Can you work these out from the model? Positions are in its coordinate system, mm. A direction names the side the tool comes from. Round coordinates to 2 decimals unless told otherwise and drop trailing zeros. Loops run counter-clockwise (first coordinate to the right, second up) from the corner with the lowest first, then second, coordinate; pieces in that order, holes last. Notation, with made-up numbers: M -13.75,20 L 31.25,20 A23 cw 31.25,31 Z; hole C 89,65 d6. An arc over 180 degrees is marked long. Use a Markdown table: item, result. Add a question column.
```python
from build123d import *

# Parameters (mm, degrees)
SKETCH1_R           = 3
SKETCH1_R_2         = 1.6
BOSS_EXTRUDE1_DEPTH = 3


with BuildPart() as part:
    # Sketch1 → Boss-Extrude1 (new body)
    with BuildSketch(Plane.XY):
        Polygon((330.61212976, -150), (350.61212976, -150), (350.61212976, -193), (345.61212976, -198), (330.61212976, -198), (308.61212976, -198), (303.61212976, -193), (303.61212976, -187), (308.61212976, -182), (325.61212976, -182), (330.61212976, -177), align=None)
        with Locations((311.11212976, -187.1)):
            Circle(SKETCH1_R, mode=Mode.SUBTRACT)
        with Locations((334.61212976, -155)):
            Circle(SKETCH1_R_2, mode=Mode.SUBTRACT)
        with Locations((346.61212976, -155)):
            Circle(SKETCH1_R_2, mode=Mode.SUBTRACT)
        with Locations((334.61212976, -175)):
            Circle(SKETCH1_R_2, mode=Mode.SUBTRACT)
        with Locations((346.61212976, -175)):
            Circle(SKETCH1_R_2, mode=Mode.SUBTRACT)
    extrude(amount=BOSS_EXTRUDE1_DEPTH)


solid = part.part
```
(1) Suppose I cut it at A-A on y = -155. List the corners of the cut face in (x, z) for me, and give its area (3 significant figures).
(2) If I drill on probe 1 along X at (y, z) = (-155, 0.7); probe 2 along Y at (x, z) = (334, 1.9); probe 3 along X at (y, z) = (-187.1, 0.9), over which ranges is the centre line in solid material (lowest first)? Write a range as [from, to].
(3) Thinking about a two-plate mould opening in X: for faces 1 (the face through (330.612, -164, 1)), 2 (the face through (327, -198, 1)), 3 (the face through (335.35, -176.42, 1.48)), which applies, released by +X, released by -X, zero draft, split by the parting line, or undercut?
(4) Suppose I cut it at C-C on x = 310. List the corners of the cut face in (y, z) for me, and give its area (3 significant figures).
(5) Suppose I cut it at D-D on x = 319.5. List the corners of the cut face in (y, z) for me, and give its area (3 significant figures).
(6) On a 3-axis mill with a long thin cutter (end or side, diameter ignored), from which of +Z, -Z, +X, -X, +Y, -Y can I reach the whole of each face in a straight line? I mean faces 4 (the face through (317, -182, 1)), 5 (the face through (335.35, -156.42, 1.48)). Say none if no direction works.
(7) Suppose I cut it at B-B on z = 1.3. List the corners of the cut face in (x, y) for me, and give its area (3 significant figures).
(8) I'm going to push flat-ended pins straight in: pin 1 (1.9 mm diameter, centred on x = 346.61, y = -175, fed in from +Z); pin 2 (1.5 mm diameter, centred on x = 316.5, z = 1.5, fed in from +Y). Where does each tip first touch, or does it pass through?
Results below:
| question | item | result |
|---|---|---|
| 1 | outline | M 330.61,0 L 333.01,0 L 333.01,3 L 330.61,3 Z; M 336.21,0 L 345.01,0 L 345.01,3 L 336.21,3 Z; M 348.21,0 L 350.61,0 L 350.61,3 L 348.21,3 Z |
| 1 | area | 40.8 mm² |
| 2 | probe 1 | x = [330.61, 333.01], [336.21, 345.01], [348.21, 350.61] |
| 2 | probe 2 | y = [-198, -176.48], [-173.52, -156.48], [-153.52, -150] |
| 2 | probe 3 | x = [303.61, 308.11], [314.11, 350.61] |
| 3 | face 1 | released by -X |
| 3 | face 2 | zero draft |
| 3 | face 3 | undercut |
| 4 | outline | M -198,0 L -189.89,0 L -189.89,3 L -198,3 Z; M -184.31,0 L -182,0 L -182,3 L -184.31,3 Z |
| 4 | area | 31.3 mm² |
| 5 | outline | M -198,0 L -182,0 L -182,3 L -198,3 Z |
| 5 | area | 48.0 mm² |
| 6 | face 4 | +Z, -Z, -X, +Y |
| 6 | face 5 | +Z, -Z |
| 7 | outline | M 303.61,-193 L 308.61,-198 L 345.61,-198 L 350.61,-193 L 350.61,-150 L 330.61,-150 L 330.61,-177 L 325.61,-182 L 308.61,-182 L 303.61,-187 Z; hole C 311.11,-187.1 d6; hole C 334.61,-175 d3.2; hole C 334.61,-155 d3.2; hole C 346.61,-175 d3.2; hole C 346.61,-155 d3.2 |
| 7 | area | 1,310 mm² |
| 8 | pin 1 | passes through |
| 8 | pin 2 | stops at y = -182 |
